```python
from build123d import *

# Parameters (mm, degrees)
BOSS_EXTRUDE1_DEPTH     = 3.75
BOSS_EXTRUDE3_DEPTH     = 3
SKETCH8_W               = 47.9125
SKETCH8_H               = 1.5
BOSS_EXTRUDE5_DEPTH     = 2
FILLET4_R               = 2
CUT_EXTRUDE1_DEPTH      = 127.75665663
CUT_EXTRUDE1_DEPTH_BACK = 4
SKETCH9_W               = 50
SKETCH9_H               = 1.55
CUT_EXTRUDE2_DEPTH      = 1.05
FILLET6_R               = 1
CHAMFER1_SIZE           = 5


with BuildPart() as part:
    # Sketch1 → Boss-Extrude1 (new, symmetric)
    with BuildSketch(Plane(origin=(0, 0, 0), x_dir=(1, 0, 0), z_dir=(0, 1, 0))):
        Polygon((-125, -10), (125, -10), (105, 10), (-105, 10), align=None)
    extrude(amount=BOSS_EXTRUDE1_DEPTH, both=True)

    # Sketch3 → Boss-Extrude3 (add)
    with BuildSketch(Plane(origin=(0, 2.75, 0), x_dir=(-1, 0, 0), z_dir=(0, 1, 0))):
        Polygon((-69.20625, 20), (-30.79375, 20), (-30.79375, 13), (-26.04375, 13), (-26.04375, 10), (-73.95625, 10), (-73.95625, 13), (-69.20625, 13), align=None)
    extrude(amount=-BOSS_EXTRUDE3_DEPTH)

    # Sketch8 → Boss-Extrude5 (add)
    with BuildSketch(Plane.XZ.offset(0.25)):
        with Locations((50, 10.75)):
            Rectangle(SKETCH8_W, SKETCH8_H)
    extrude(amount=BOSS_EXTRUDE5_DEPTH)

    # Fillet4
    fillet4_edges = [part.edges().sort_by_distance(p)[0] for p in [
        (30.79375, 1.25, 13),
        (69.20625, 1.25, 13),
    ]]
    fillet(fillet4_edges, radius=FILLET4_R)

    # Sketch4 → Cut-Extrude1 (cut, two sides: drawn at the far end of the back side and taken through both)
    with BuildSketch(Plane(origin=(0, 2.75, 0), x_dir=(-1, 0, 0), z_dir=(0, 1, 0)).offset(-CUT_EXTRUDE1_DEPTH_BACK)):
        Polygon((22, 0), (78, 0), (78, 5), (75, 5), (75, 10), (25, 10), (25, 5), (22, 5), align=None)
    extrude(amount=CUT_EXTRUDE1_DEPTH + CUT_EXTRUDE1_DEPTH_BACK, mode=Mode.SUBTRACT)

    # Sketch9 → Cut-Extrude2 (cut)
    with BuildSketch(Plane(origin=(0, -1.25, 0), x_dir=(1, 0, 0), z_dir=(0, 1, 0))):
        with Locations((-50, -9.225)):
            Rectangle(SKETCH9_W, SKETCH9_H)
    extrude(amount=-CUT_EXTRUDE2_DEPTH, mode=Mode.SUBTRACT)

    # Fillet6
    fillet6_edges = [part.edges().sort_by_distance(p)[0] for p in [
        (-75, 1.25, 5),
        (-22, 1.25, 0),
        (-78, 1.25, 0),
        (-78, 1.25, 5),
        (-25, 1.25, 5),
        (-22, 1.25, 5),
    ]]
    fillet(fillet6_edges, radius=FILLET6_R)

    # Chamfer1
    chamfer1_edges = [part.edges().sort_by_distance(p)[0] for p in [
        (0, -3.75, -10),
    ]]
    chamfer(chamfer1_edges, length=CHAMFER1_SIZE)


solid = part.part
```
For this review, take the finished solid that the model builds, in its own axes (mm). A direction names the side the tool comes from. Coordinates: 2 decimals unless noted, no trailing zeros. Write each loop counter-clockwise with the first axis right and the second up, starting at its lowest first coordinate (ties: lowest second). Pieces come first, ordered by that corner, then holes. Notation, with made-up numbers: (31, -25.75) - (83, -25.75) arc R27 cw to (83, -7.75) - close; hole circle Ø10 at (17.5, 4.5). An arc over 180 degrees is marked (long way). Answer in a Markdown table with one row per item. Add a question column.
Q1. Tool access review of faces 5 (the flat face through (50, -0.25, 16)), 6 (the flat face through (-2, -3.75, 2)): name each direction out of +Z, -Z, +X, -X, +Y, -Y from which nothing blocks a thin tool from reaching the whole face with its end or side.
Q2. We need section A-A, the plane x = 36. State the section outline as (y, z) points, and give its area (4 significant figures).
Q3. We need section B-B, the plane x = -43.5. State the section outline as (y, z) points, and give its area (3 significant figures).
Q4. For P1, Ø4, axis at x = 8.5, y = -1.5, coming from the -Z side; P2, Ø0.5, axis at x = -23.5, y = 0.5, coming from the -Z side; P3, Ø1.2, axis at y = -0.5, z = 7, coming from the -X side, all flat-tipped, find the tip position at first contact; note any pin that passes through.
Q5. For probe 1 along Y at (x, z) = (-47.5, 2); probe 2 along Y at (x, z) = (39.5, 16); probe 3 along X at (y, z) = (0.75, 19), list the stretches that pass through material, from the lowest coordinate up.
Q6. Draft analysis for pull direction X (two halves, no side actions). For faces 1 (the flat face through (-75, 1, 8)), 2 (the flat face through (-115, 0, 0)), 3 (the flat face through (50, 2.75, 15)), 4 (the flat face through (-25, 1, 8)), state which applies: +X half, -X half, draft (parallel to the pull), parting line (faces both ways), or undercut.
Q7. We need section C-C, the plane x = 79. State the section outline as (y, z) points, and give its area (4 significant figures).
Answer list:
| question | item | result |
|---|---|---|
| 1 | face 5 | +Z, +X, -X, -Y |
| 1 | face 6 | +Z, -Z, +X, -X, -Y |
| 2 | outline | (-3.75, -5) - (1.25, -10) - (3.75, -10) - (3.75, 10) - (2.75, 10) - (2.75, 20) - (-0.25, 20) - (-0.25, 11.5) - (-2.25, 11.5) - (-2.25, 10) - (-3.75, 10) - close |
| 2 | area | 170.5 mm2 |
| 3 | outline | (-3.75, -5) - (1.25, -10) - (3.75, -10) - (3.75, 0) - (-1.25, 0) - (-1.25, 8.45) - (-2.3, 8.45) - (-2.3, 10) - (-3.75, 10) - close |
| 3 | area | 85.9 mm2 |
| 4 | P1 | stops at z = -9.25 |
| 4 | P2 | stops at z = -9.5 |
| 4 | P3 | stops at x = -122.6 |
| 5 | probe 1 | y = -3.75 to -1.25 |
| 5 | probe 2 | y = -0.25 to 2.75 |
| 5 | probe 3 | x = 30.79 to 69.21 |
| 6 | face 1 | undercut |
| 6 | face 2 | -X half |
| 6 | face 3 | draft |
| 6 | face 4 | undercut |
| 7 | outline | (-3.75, -5) - (1.25, -10) - (3.75, -10) - (3.75, 10) - (-3.75, 10) - close |
| 7 | area | 137.5 mm2 |
